Source: CAD feature listing. Evaluate the final solid. Frame: model axes, mm. A direction names the side the tool comes from. Coordinates: 2 decimals unless noted, no trailing zeros. Order: outer loops, then holes, each group sorted by start corner. A loop starts at its lowest first (then second) coordinate and runs counter-clockwise, first axis right, second up. Notation, with made-up numbers: (71, 14) -> (108, 14) arc R27 ccw to (108, 39) -> close; hole circle Ø10 at (-26, -15.75). An arc over 180 degrees is marked (long way). Write item = value, one per line. Start each with the question number.
Item 1: Section query C-C (x = 21). Output: boundary loops of the cut face in (y, z), then the cut area to 3 significant figures.
Item 2: Set-up query: faces 1 (the cylindrical face through (14.084, 3.173, -0.705)), 2 (the flat face through (27, 3.92, -1.42)), 3 (the cylindrical face through (7.305, -9.81, 1.532)). Return all of +Z, -Z, +X, -X, +Y, -Y with unobstructed straight access to the full face (end or side cutting, diameter ignored); none if empty.
Item 3: Section query B-B (y = 0). Output: boundary loops of the cut face in (x, z).
Item 4: Ray query, line 1 along Y through (x, z) = (3.75, 0); line 2 along X through (y, z) = (-5.75, 0); line 3 along Y through (x, z) = (16, 0). Return the intervals inside material, ascending. Write a range as [from, to].
Item 5: Section query A-A (z = 0). Count the separate pieces of the cut face and the enclosed holes in it, then the cut area to 3 significant figures.
Item 6: Section query D-D (y = -10.25). Output: boundary loops of the cut face in (x, z).
Item 7: Contact query for flat-ended pins moving along their axis: pin 1 (3 mm diameter, centred on y = 0.5, z = -4.5, fed in from -X); pin 2 (1.5 mm diameter, centred on x = 33, z = -2.5, fed in from -Y); pin 3 (2 mm diameter, centred on x = 19, z = 1.5, fed in from -Y); pin 4 (4 mm diameter, centred on y = 0, z = 0, fed in from -X). Output: stop coordinate, or through.
Item 8: Mould query, pull axis Z, two halves, no side actions, for faces 4 (the cylindrical face through (35.112, 3.905, -0.867)), 5 (the cylindrical face through (10.399, -8.694, -1.908)), 6 (the flat face through (20, -1.5, 0.7)), 7 (the flat face through (13, -15, -1)). Classes: released by +Z, released by -Z, zero draft, split by the parting line, or undercut.
Autodesk Inventor part; units mm, degrees
ref_plane "Work Plane1" through (13.5, -6, 0) normal (0, 1, 0) x (-1, 0, 0)
ref_plane "YZ Plane" through (0, 0, 0) normal (1, 0, 0) x (0, 1, 0)
ref_plane "XY Plane" through (0, 0, 0) normal (0, 0, 1) x (1, 0, 0)
sketch "Sketch1" plane through (0, 0, 0) normal (0, 1, 0) x (-1, 0, 0)
  line L0 (0, 0) -> (-52, 0)
  line L1 (0, 4) -> (-8, 4)
  line L2 (0, 6) -> (-27, 6)
  line L3 (0, 0) -> (0, 37) construction
  line L4 (-8, 3.25) -> (-20, 3.25)
  line L5 (-8, 4) -> (-8, 3.25)
  line L6 (-20, 1.5) -> (-27, 1.5)
  line L7 (-20, 3.25) -> (-20, 1.5)
  line L8 (-27, 6) -> (-27, 4)
  line L9 (-27, 4) -> (-43, 4)
  line L10 (-34, 2) -> (-43, 2)
  line L11 (-43, 4) -> (-43, 2)
  line L12 (-34, 2) -> (-34, 1.5)
  line L13 (-34, 1.5) -> (-27, 1.5)
  line L14 (0, 6) -> (0, 4)
  point P0 (-8, 3.625)
  dimension "d0" = 8
  dimension "d1" = 12
  dimension "d2" = 27
  dimension "d3" = 6.5
  dimension "d4" = 8
  dimension "d5" = 20
  dimension "d6" = 3
  dimension "d7" = 8
  dimension "d8" = 16
  dimension "d9" = 4
  dimension "d10" = 9
revolve "Revolution1" add sketch "Sketch1" angle 360 about axis through (0, 0, 0) along (1, 0, 0)
thread "Thread1"
thread "Thread2"
ref_plane "Work Plane1" through (13.5, -6, 0) normal (0, 1, 0) x (-1, 0, 0)
sketch "Sketch2" plane through (13.5, -6, 0) normal (0, 1, 0) x (-1, 0, 0)
  circle A0 centre (2.5, 0) radius 4
  line L0 (13.5, 6) -> (13.5, -6)
  line L1 (13.5, 0) -> (-13.5, 0)
  line L2 (-13.5, 6) -> (-13.5, -6)
  dimension "d16" = 8
  dimension "d17" = 7
extrude "Extrusion1" add sketch "Sketch2" against normal blind 9
sketch "Sketch3" plane through (11, -15, 0) normal (0, -1, 0) x (1, 0, 0)
  circle A0 centre (0, 0) radius 4
  point P0 (-11, 0)
extrude "Extrusion2" add sketch "Sketch2" along normal blind 2
hole "Hole2" at (11, -15, 0) direction (0, 1, 0) diameter 4 end up to surface
properties part number "HUDSON-1-81"
Computed:
q1.outline = circle Ø12 at (0, 0); hole circle Ø3 at (0, 0)
q1.area = 106 mm^2
q2.face_1 = -X
q2.face_2 = +X
q2.face_3 = -Y
q3.outline = (0, -6) -> (27, -6) -> (27, -4) -> (43, -4) -> (43, -2) -> (34, -2) -> (34, -1.5) -> (20, -1.5) -> (20, -3.25) -> (8, -3.25) -> (8, -4) -> (0, -4) -> close; (0, 4) -> (8, 4) -> (8, 3.25) -> (20, 3.25) -> (20, 1.5) -> (34, 1.5) -> (34, 2) -> (43, 2) -> (43, 4) -> (27, 4) -> (27, 6) -> (0, 6) -> close
q4.line_1 = [-6, -4], [4, 6]
q4.line_2 = [0, 9], [13, 27]
q4.line_3 = [-6, -3.25], [3.25, 6]
q5.separate_pieces = 3
q5.enclosed_holes = 0
q5.area = 257 mm^2
q6.outline = circle Ø8 at (11, 0); hole circle Ø4 at (11, 0)
q7.pin_1 = 0
q7.pin_2 = -3.6
q7.pin_3 = -5.98
q7.pin_4 = 20
q8.face_4 = split by the parting line
q8.face_5 = undercut
q8.face_6 = undercut
q8.face_7 = zero draft
